Part model, mm, in its own coordinate system. A direction names the side the tool comes from. Coordinates: 2 decimals unless noted, no trailing zeros. Order: outer loops, then holes, each group sorted by start corner. A loop starts at its lowest first (then second) coordinate and runs counter-clockwise, first axis right, second up.
1) Mould opens along X. For faces 1 (the cylindrical face through (1.522, 1.565, -86.633)), 2 (the cylindrical face through (-151.74, 1.57, -60.7)), 3 (the flat face through (3, 3.175, -2)) say: +X half, -X half, draft (parallel to the pull), parting line (faces both ways), or undercut.
2) Cut at C-C (y = 1.1). Give the number of separate pieces and of enclosed holes in the cut face, and give its area (3 significant figures).
3) Pin check, flat tip, straight feed: pin 1 Ø2.5 at (x, z) = (165.1, 104.775) entering from -Y. Stop position of the tip, or through.
4) Cut at D-D (x = -4). List the corners of the cut face in (y, z) (3 decimals).
5) Cut at B-B (z = -78). List the corners of the cut face in (x, y) (3 decimals), and give its area (3 significant figures).
6) Wall check: L1, parallel to Z at x = -55, y = 1.85; L2, parallel to X at y = 0.7, z = 0; L3, parallel to X at y = 2.5, z = 56. Give the ranges that are in metal, low to high.
7) Tool access for faces 4 (the flat face through (3, 0, -2)), 5 (the flat face through (176, 1.651, -1)): list every direction of +Z, -Z, +X, -X, +Y, -Y with a clear straight run to the whole face (end or side of a thin tool).
8) Cut at A-A (x = -119.38). List the corners of the cut face in (y, z) (3 decimals), and give its area (3 significant figures).
```python
from build123d import *

# Parameters (mm, degrees)
SKETCH1_R           = 33.147
SKETCH1_R_2         = 2.2479
BOSS_EXTRUDE1_DEPTH = 3.175
CUT_EXTRUDE1_DEPTH  = 1.524


with BuildPart() as part:
    # Sketch1 → Boss-Extrude1 (new body)
    with BuildSketch(Plane(origin=(0, 0, 0), x_dir=(1, 0, 0), z_dir=(0, 1, 0))):
        with BuildLine():
            Line((-180.975, 114.3), (180.975, 114.3))
            ThreePointArc((180.975, 114.3), (183.22006403, 113.37006403), (184.15, 111.125))
            Line((184.15, 111.125), (184.15, -111.125))
            ThreePointArc((184.15, -111.125), (183.22006403, -113.37006403), (180.975, -114.3))
            Line((180.975, -114.3), (-180.975, -114.3))
            ThreePointArc((-180.975, -114.3), (-183.22006403, -113.37006403), (-184.15, -111.125))
            Line((-184.15, -111.125), (-184.15, 111.125))
            ThreePointArc((-184.15, 111.125), (-183.22006403, 113.37006403), (-180.975, 114.3))
        make_face()
        with Locations(Location((119.508581684, -53.5178, 0), (0, 0, 270))):
            Circle(SKETCH1_R, mode=Mode.SUBTRACT)
        with Locations(Location((165.1, 0, 0), (0, 0, 270))):
            Circle(SKETCH1_R_2, mode=Mode.SUBTRACT)
        with Locations(Location((-171.45, 0, 0), (0, 0, 270))):
            Circle(SKETCH1_R_2, mode=Mode.SUBTRACT)
        with Locations(Location((-55.033333333, 0, 0), (0, 0, 270))):
            Circle(SKETCH1_R_2, mode=Mode.SUBTRACT)
        with Locations(Location((55.033333333, 0, 0), (0, 0, 270))):
            Circle(SKETCH1_R_2, mode=Mode.SUBTRACT)
        with Locations(Location((119.508581684, 53.5178, 0), (0, 0, 270))):
            Circle(SKETCH1_R, mode=Mode.SUBTRACT)
        with Locations(Location((0.064290842, 53.5178, 0), (0, 0, 270))):
            Circle(SKETCH1_R, mode=Mode.SUBTRACT)
        with Locations(Location((0.064290842, -53.5178, 0), (0, 0, 270))):
            Circle(SKETCH1_R, mode=Mode.SUBTRACT)
        with Locations(Location((-119.38, 53.5178, 0), (0, 0, 270))):
            Circle(SKETCH1_R, mode=Mode.SUBTRACT)
        with Locations(Location((-119.38, -53.5178, 0), (0, 0, 270))):
            Circle(SKETCH1_R, mode=Mode.SUBTRACT)
        with Locations(Location((-149.225, -104.775, 0), (0, 0, 270))):
            Circle(SKETCH1_R_2, mode=Mode.SUBTRACT)
        with Locations(Location((-55.033333333, -104.775, 0), (0, 0, 270))):
            Circle(SKETCH1_R_2, mode=Mode.SUBTRACT)
        with Locations(Location((55.033333333, -104.775, 0), (0, 0, 270))):
            Circle(SKETCH1_R_2, mode=Mode.SUBTRACT)
        with Locations(Location((165.1, -104.775, 0), (0, 0, 270))):
            Circle(SKETCH1_R_2, mode=Mode.SUBTRACT)
        with Locations(Location((-149.225, 104.775, 0), (0, 0, 270))):
            Circle(SKETCH1_R_2, mode=Mode.SUBTRACT)
        with Locations(Location((-55.033333333, 104.775, 0), (0, 0, 270))):
            Circle(SKETCH1_R_2, mode=Mode.SUBTRACT)
        with Locations(Location((55.033333333, 104.775, 0), (0, 0, 270))):
            Circle(SKETCH1_R_2, mode=Mode.SUBTRACT)
        with Locations(Location((165.1, 104.775, 0), (0, 0, 270))):
            Circle(SKETCH1_R_2, mode=Mode.SUBTRACT)
    extrude(amount=BOSS_EXTRUDE1_DEPTH)

    # Sketch2 → Cut-Extrude1 (cut)
    with BuildSketch(Plane(origin=(0, 3.175, 0), x_dir=(1, 0, 0), z_dir=(0, 1, 0))):
        with BuildLine():
            Line((171.45, 3.35692423), (179.668619792, 5.426396401))
            Line((179.668619792, 5.426396401), (179.668619792, 4.229494039))
            Line((179.668619792, 4.229494039), (174.263626046, 3.009542664))
            add(Edge.make_bspline(
                [(174.263626046, 3.009542664), (173.984868687, 2.946317196), (173.430199851, 2.82051174), (172.875222779, 2.696073098), (172.599157976, 2.63417301)],
                knots=[0, 0, 0, 0, 1.00513078, 2, 2, 2, 2], degree=3))
            add(Edge.make_bspline(
                [(172.599157976, 2.63417301), (172.698424046, 2.604865261), (172.8858203, 2.549537571), (173.151472547, 2.474745256), (173.383326442, 2.406813793), (173.582462852, 2.348939672), (173.749161553, 2.302079221), (173.881374159, 2.261620439), (173.981689825, 2.234044239), (174.036994185, 2.217702533), (174.059477638, 2.21105897)],
                knots=[0, 0, 0, 0, 1.633809233, 3.084334118, 4.356383392, 5.447555203, 6.357852567, 7.089694452, 7.629924063, 8, 8, 8, 8], degree=3))
            Line((174.059477638, 2.21105897), (179.668619792, 0.587749853))
            Line((179.668619792, 0.587749853), (179.668619792, -0.806715484))
            Line((179.668619792, -0.806715484), (175.551078105, -1.980568832))
            add(Edge.make_bspline(
                [(175.551078105, -1.980568832), (175.296712529, -2.045349191), (174.795158662, -2.173082039), (174.048075598, -2.342795744), (173.319116921, -2.49943607), (172.836990124, -2.589663839), (172.599157976, -2.63417301)],
                knots=[0, 0, 0, 0, 1.04154457, 2.053700482, 3.039894486, 4, 4, 4, 4], degree=3))
            add(Edge.make_bspline(
                [(172.599157976, -2.63417301), (172.720980898, -2.661645998), (172.977226876, -2.719433502), (173.381816931, -2.809933441), (173.825093055, -2.910447181), (174.134101714, -2.979956246), (174.294906851, -3.016128097)],
                knots=[0, 0, 0, 0, 0.862132589, 1.813435466, 2.862132822, 4, 4, 4, 4], degree=3))
            Line((174.294906851, -3.016128097), (179.668619792, -4.229494039))
            Line((179.668619792, -4.229494039), (179.668619792, -5.426396401))
            Line((179.668619792, -5.426396401), (171.45, -3.355277872))
            Line((171.45, -3.355277872), (171.45, -2.080996678))
            Line((171.45, -2.080996678), (177.730856271, -0.363845147))
            add(Edge.make_bspline(
                [(177.730856271, -0.363845147), (177.792257478, -0.346602472), (177.908896909, -0.31384781), (178.075345329, -0.27091412), (178.221729866, -0.228338076), (178.349942301, -0.194473031), (178.458690649, -0.165165669), (178.547656515, -0.139212748), (178.618581103, -0.122520526), (178.658892529, -0.110449487), (178.675865838, -0.10536692)],
                knots=[0, 0, 0, 0, 1.562239628, 2.967673567, 4.210417925, 5.296319877, 6.215971374, 6.969386481, 7.566055473, 8, 8, 8, 8], degree=3))
            add(Edge.make_bspline(
                [(178.675865838, -0.10536692), (178.568229296, -0.074892118), (178.364849129, -0.017309719), (178.078532422, 0.067967153), (177.826773257, 0.139523409), (177.671018148, 0.184870245), (177.599147621, 0.205794766)],
                knots=[0, 0, 0, 0, 1.197730334, 2.263121701, 3.198547257, 4, 4, 4, 4], degree=3))
            Line((177.599147621, 0.205794766), (171.45, 1.985507906))
            Line((171.45, 1.985507906), (171.45, 3.35692423))
        make_face()
    extrude(amount=-CUT_EXTRUDE1_DEPTH, mode=Mode.SUBTRACT)


solid = part.part
```
Geometry check:
1. face 1: undercut
1. face 2: undercut
1. face 3: draft
2. separate pieces: 1
2. enclosed holes: 18
2. area: 63,300 mm2
3. pin 1: passes through
4. outline: (0, -114.3) - (3.175, -114.3) - (3.175, -86.415) - (0, -86.415) - close; (0, -20.621) - (3.175, -20.621) - (3.175, 20.621) - (0, 20.621) - close; (0, 86.415) - (3.175, 86.415) - (3.175, 114.3) - (0, 114.3) - close
5. outline: (-184.15, 0) - (-141.726, 0) - (-141.726, 3.175) - (-184.15, 3.175) - close; (-97.034, 0) - (-22.282, 0) - (-22.282, 3.175) - (-97.034, 3.175) - close; (22.41, 0) - (97.163, 0) - (97.163, 3.175) - (22.41, 3.175) - close; (141.855, 0) - (184.15, 0) - (184.15, 3.175) - (141.855, 3.175) - close
5. area: 744 mm2
6. L1: z = -114.3 to -107.02, -102.53 to -2.25, 2.25 to 102.53, 107.02 to 114.3
6. L2: x = -184.15 to -173.7, -169.2 to -57.28, -52.79 to 52.79, 57.28 to 162.85, 167.35 to 184.15
6. L3: x = -184.15 to -152.43, -86.33 to -32.99, 33.12 to 86.45, 152.56 to 184.15
7. face 4: +Z, -Z, +X, -X, -Y
7. face 5: +Y
8. outline: (0, -114.3) - (3.175, -114.3) - (3.175, -86.665) - (0, -86.665) - close; (0, -20.371) - (3.175, -20.371) - (3.175, 20.371) - (0, 20.371) - close; (0, 86.665) - (3.175, 86.665) - (3.175, 114.3) - (0, 114.3) - close
8. area: 305 mm2
